```python
from build123d import *

# Parameters (mm, degrees)
SKETCH_1_W                   = 10
SKETCH_1_H                   = 75
EXTRUDE_2_DEPTH              = 20
SKETCH_10_W                  = 31
SKETCH_10_H                  = 5
EXTRUDE_3_DEPTH              = 70
SKETCH_11_W                  = 5
SKETCH_11_H                  = 18
EXTRUDE_4_DEPTH              = 70
SKETCH_12_W                  = 5
SKETCH_12_H                  = 18
EXTRUDE_5_DEPTH              = 70
SKETCH_13_W                  = 60
SKETCH_13_H                  = 8
CUT_EXTRUDE_6_DEPTH          = 20
SKETCH_14_W                  = 10
SKETCH_14_H                  = 3.5
CUT_EXTRUDE_7_DEPTH          = 20
HOLE_WIZARD_M3_1_D           = 3.4
HOLE_WIZARD_M3_1_DEPTH       = 20
HOLE_WIZARD_M3_1_CBORE_D     = 6.7
HOLE_WIZARD_M3_1_CBORE_DEPTH = 1.65
HOLE_WIZARD_M3_1_TIP         = 1.021463052
CUT_EXTRUDE_8_DEPTH          = 2.5
CUT_EXTRUDE_9_DEPTH          = 5


with BuildPart() as part:
    # 草图1 → 凸台-拉伸2 (new body)
    with BuildSketch(Plane(origin=(0, 0, 0), x_dir=(1, 0, 0), z_dir=(0, 1, 0))):
        with Locations((5, 37.5)):
            Rectangle(SKETCH_1_W, SKETCH_1_H)
    extrude(amount=EXTRUDE_2_DEPTH)

    # 草图10 → 凸台-拉伸3 (add)
    with BuildSketch(Plane.ZY):
        with Locations((-37.5, 2.5)):
            Rectangle(SKETCH_10_W, SKETCH_10_H)
    extrude(amount=EXTRUDE_3_DEPTH)

    # 草图11 → 凸台-拉伸4 (add)
    with BuildSketch(Plane.ZY):
        with Locations((-19.5, 9)):
            Rectangle(SKETCH_11_W, SKETCH_11_H)
    extrude(amount=EXTRUDE_4_DEPTH)

    # 草图12 → 凸台-拉伸5 (add)
    with BuildSketch(Plane.ZY):
        with Locations((-55.5, 9)):
            Rectangle(SKETCH_12_W, SKETCH_12_H)
    extrude(amount=EXTRUDE_5_DEPTH)

    # 草图13 → 切除-拉伸6 (cut)
    with BuildSketch(Plane(origin=(0, 5, 0), x_dir=(1, 0, 0), z_dir=(0, 1, 0))):
        with Locations((-40, 37.5)):
            Rectangle(SKETCH_13_W, SKETCH_13_H)
    extrude(amount=-CUT_EXTRUDE_6_DEPTH, mode=Mode.SUBTRACT)

    # 草图14 → 切除-拉伸7 (cut)
    with BuildSketch(Plane(origin=(0, 5, 0), x_dir=(1, 0, 0), z_dir=(0, 1, 0))):
        with Locations((-18, 43.25)):
            Rectangle(SKETCH_14_W, SKETCH_14_H)
    extrude(amount=-CUT_EXTRUDE_7_DEPTH, mode=Mode.SUBTRACT)

    # M3 凹圆头螺钉的柱形沉头孔1
    with Locations(Plane(origin=(0, 10, -37.5), x_dir=(0, 0, -1), z_dir=(-1, 0, 0))):
        with Locations((0, 0)):
            CounterBoreHole(HOLE_WIZARD_M3_1_D / 2, HOLE_WIZARD_M3_1_CBORE_D / 2, HOLE_WIZARD_M3_1_CBORE_DEPTH, depth=HOLE_WIZARD_M3_1_DEPTH)
            with Locations((0, 0, -(HOLE_WIZARD_M3_1_DEPTH + HOLE_WIZARD_M3_1_TIP / 2))):  # 118° drill point
                Cone(0, HOLE_WIZARD_M3_1_D / 2, HOLE_WIZARD_M3_1_TIP, mode=Mode.SUBTRACT)

    # 草图5 → 切除-拉伸8 (cut)
    with BuildSketch(Plane(origin=(10, 0, 0), x_dir=(0, 0, -1), z_dir=(1, 0, 0))):
        with BuildLine():
            Line((63.5, 14.5), (39.054281703, 17.132615817))
            ThreePointArc((39.054281703, 17.132615817), (43.184903536, 14.579505626), (44.8, 10))
            ThreePointArc((44.8, 10), (43.184903536, 5.420494374), (39.054281703, 2.867384183))
            Line((39.054281703, 2.867384183), (63.5, 5.5))
            ThreePointArc((63.5, 5.5), (68, 10), (63.5, 14.5))
        make_face()
        with BuildLine():
            Line((37.5, 17.3), (35.945718297, 17.132615817))
            ThreePointArc((35.945718297, 17.132615817), (30.2, 10), (35.945718297, 2.867384183))
            Line((35.945718297, 2.867384183), (37.5, 2.7))
            Line((37.5, 2.7), (39.054281703, 2.867384183))
            ThreePointArc((39.054281703, 2.867384183), (43.184903536, 5.420494374), (44.8, 10))
            ThreePointArc((44.8, 10), (43.184903536, 14.579505626), (39.054281703, 17.132615817))
            Line((39.054281703, 17.132615817), (37.5, 17.3))
        make_face()
        with BuildLine():
            Line((35.945718297, 17.132615817), (11.5, 14.5))
            ThreePointArc((11.5, 14.5), (7, 10), (11.5, 5.5))
            Line((11.5, 5.5), (35.945718297, 2.867384183))
            ThreePointArc((35.945718297, 2.867384183), (30.2, 10), (35.945718297, 17.132615817))
        make_face()
    extrude(amount=-CUT_EXTRUDE_8_DEPTH, mode=Mode.SUBTRACT)

    # 草图16 → 切除-拉伸9 (cut)
    with BuildSketch(Plane(origin=(10, 0, 0), x_dir=(0, 0, -1), z_dir=(1, 0, 0))):
        Polygon((37.5, 17.3), (25.568986317, 16.015121603), (25.568986317, 3.984878397), (37.5, 2.7), (49.431013683, 3.984878397), (49.431013683, 16.015121603), align=None)
    extrude(amount=-CUT_EXTRUDE_9_DEPTH, mode=Mode.SUBTRACT)


solid = part.part
```
Input: part model. Units: mm. Frame: model coordinates. A direction names the side the tool comes from. Coordinates: 2 decimals unless noted, no trailing zeros. Write each loop counter-clockwise with the first axis right and the second up, starting at its lowest first coordinate (ties: lowest second). Pieces come first, ordered by that corner, then holes. Notation, with made-up numbers: (17.5, -34.75) -> (26.5, -34.75) arc R21 ccw to (26.5, -25.75) -> close; hole circle Ø2 at (84, 40). An arc over 180 degrees is marked (long way). Answer as a JSON object with one key per item and string values.
1. Access query for faces 4 (the face through (-40, 3, -33.5)), 5 (the face through (9, 10, -7)), 6 (the face through (-35, 9, -58)), 7 (the face through (-13, 3, -43)), 8 (the face through (-35, 5, -31)). Directions: +Z, -Z, +X, -X, +Y, -Y. A direction counts if a zero-diameter tool reaches every point of the face in a straight line with its end or side. Return the directions, or none.
Result set:
{"face 4": "-X, +Y, -Y", "face 5": "+X", "face 6": "-Z, -X, +Y, -Y", "face 7": "+Y, -Y", "face 8": "-X, +Y"}
2. Section B-B on y = 10. Return the cut outline in (x, z), then the cut area to 3 significant figures.
Result set:
{"outline": "(-70, -58) -> (0, -58) -> (0, -75) -> (10, -75) -> (10, -68) -> (7.5, -68) -> (7.5, -49.43) -> (5, -49.43) -> (5, -39.2) -> (1.65, -39.2) -> (1.65, -40.85) -> (0, -40.85) -> (0, -53) -> (-70, -53) -> close; (-70, -22) -> (0, -22) -> (0, -34.15) -> (1.65, -34.15) -> (1.65, -35.8) -> (5, -35.8) -> (5, -25.57) -> (7.5, -25.57) -> (7.5, -7) -> (10, -7) -> (10, 0) -> (0, 0) -> (0, -17) -> (-70, -17) -> close", "area": "1,220 mm2"}
3. Mould query, pull axis Z, two halves, no side actions, for faces 1 (the face through (-23, 3, -43)), 2 (the face through (-35, 9, -17)), 3 (the face through (-70, 7.1, -21.7)). Classes: released by +Z, released by -Z, zero draft, split by the parting line, or undercut.
Result set:
{"face 1": "undercut", "face 2": "released by +Z", "face 3": "zero draft"}
4. Material intervals for line 1 (Z direction, x = 3.7, y = 10); line 2 (Y direction, x = 2.45, z = -37.5); line 3 (Z direction, x = 0.7, y = 10), sorted ascending. Write a range as from..to.
Result set:
{"line 1": "z = -75..-39.2, -35.8..0", "line 2": "y = 0..8.3, 11.7..20", "line 3": "z = -75..-40.85, -34.15..0"}
5. Section A-A on x = -46. Return the cut outline in (y, z).
Result set:
{"outline": "(0, -58) -> (18, -58) -> (18, -53) -> (5, -53) -> (5, -41.5) -> (0, -41.5) -> close; (0, -33.5) -> (5, -33.5) -> (5, -22) -> (18, -22) -> (18, -17) -> (0, -17) -> close"}
6. First-contact query: P1, Ø10, axis at x = -62, z = -60, coming from the +Y side; P2, Ø6, axis at y = 10, z = -34, coming from the -X side; P3, Ø3, axis at x = -28, y = 8.5, coming from the +Z side. Flat tips, straight axial feed; report the tip coordinate or a pass-through.
Result set:
{"P1": "stops at y = 18", "P2": "stops at x = 0", "P3": "stops at z = -17"}
7. Section C-C on z = -50.5. Return the cut outline in (x, y).
Result set:
{"outline": "(-70, 0) -> (10, 0) -> (10, 4.1) -> (7.5, 4.1) -> (7.5, 15.9) -> (10, 15.9) -> (10, 20) -> (0, 20) -> (0, 5) -> (-70, 5) -> close"}
8. Section D-D on x = -9. Return the cut outline in (y, z).
Result set:
{"outline": "(0, -58) -> (18, -58) -> (18, -53) -> (5, -53) -> (5, -22) -> (18, -22) -> (18, -17) -> (0, -17) -> close"}
